Here's how the part is built. I have some questions about the finished solid (model axes, mm). Round coordinates to 2 decimals unless told otherwise and drop trailing zeros. Order: outer loops, then holes, each group sorted by start corner. A loop starts at its lowest first (then second) coordinate and runs counter-clockwise, first axis right, second up. Notation, with made-up numbers: (46.5, -35) -> (56.5, -35) arc R15 cw to (56.5, -9) -> close; hole circle Ø2 at (-24.5, -8.75). An arc over 180 degrees is marked (long way). Answer in a Markdown table with one row per item.
```python
from build123d import *

# Parameters (mm, degrees)
F0_R     = 1.5
F0_R_2   = 4.5
F1_DEPTH = 3


with BuildPart() as f1:
    # F0 (on Front) → F1 (new body)
    with BuildSketch(Plane.XZ):
        with BuildLine():
            Line((20, 40), (-20, 40))
            Line((-20, 40), (-20, -40))
            Line((-20, -40), (-12.7, -40))
            ThreePointArc((-12.7, -40), (0, -27.3), (12.7, -40))
            Line((12.7, -40), (20, -40))
            Line((20, -40), (20, 40))
        make_face()
        with Locations((15, -27.3)):
            Circle(F0_R, mode=Mode.SUBTRACT)
        with Locations((0, 20)):
            Circle(F0_R_2, mode=Mode.SUBTRACT)
    extrude(amount=F1_DEPTH)


solid = f1.part
```
1. Please list where these lines run through material, in increasing order: line 1 along Z through (x, y) = (0, -2.3); line 2 along Z through (x, y) = (15, -0.75); line 3 along Z through (x, y) = (11, -2.25).
Numbers:
| item | result |
|---|---|
| line 1 | z = -27.3 to 15.5, 24.5 to 40 |
| line 2 | z = -40 to -28.8, -25.8 to 40 |
| line 3 | z = -33.65 to 40 |
2. Suppose I cut it at B-B on x = 0. Write out the boundary of the cut face in (y, z).
Numbers:
| item | result |
|---|---|
| outline | (-3, -27.3) -> (0, -27.3) -> (0, 15.5) -> (-3, 15.5) -> close; (-3, 24.5) -> (0, 24.5) -> (0, 40) -> (-3, 40) -> close |
3. We'd pull the mould along Z, two halves only. Please class faces 1 (the face through (2.419, -1.479, 23.794)), 2 (the face through (0, -3, 1)), 3 (the face through (0, -1, 40)), 4 (the face through (13.5, -1.48, -27.23)): released by +Z, released by -Z, zero draft, split by the parting line, or undercut.
Numbers:
| item | result |
|---|---|
| face 1 | undercut |
| face 2 | zero draft |
| face 3 | released by +Z |
| face 4 | undercut |
4. Suppose I cut it at D-D on x = -11. Write out the boundary of the cut face in (y, z).
Numbers:
| item | result |
|---|---|
| outline | (-3, -33.65) -> (0, -33.65) -> (0, 40) -> (-3, 40) -> close |
5. Suppose I cut it at A-A on z = 20. Write out the boundary of the cut face in (x, y).
Numbers:
| item | result |
|---|---|
| outline | (-20, -3) -> (-4.5, -3) -> (-4.5, 0) -> (-20, 0) -> close; (4.5, -3) -> (20, -3) -> (20, 0) -> (4.5, 0) -> close |
6. Suppose I cut it at C-C on y = -1.25. Write out the boundary of the cut face in (x, z), then the cut area to 3 significant figures.
Numbers:
| item | result |
|---|---|
| outline | (-20, -40) -> (-12.7, -40) arc R12.7 cw to (12.7, -40) -> (20, -40) -> (20, 40) -> (-20, 40) -> close; hole circle Ø9 at (0, 20); hole circle Ø3 at (15, -27.3) |
| area | 2,880 mm2 |
